```python
from build123d import *

# Parameters (mm, degrees)
SKETCH1_W   = 75
SKETCH1_H   = 250
SKETCH2_W   = 69.969867672
SKETCH2_H   = 30
SKETCH2_H_2 = 31.89416608
SKETCH2_H_3 = 30.244467835


with BuildPart() as part:
    # Sketch1 → Revolve1 (revolve)
    with BuildSketch(Plane.XY, mode=Mode.PRIVATE) as revolve1_sk:
        with Locations((-112.5, 125)):
            Rectangle(SKETCH1_W, SKETCH1_H)
    revolve(revolve1_sk.sketch.rotate(Axis((0, 0, 0), (0, 1, 0)), 270), axis=Axis((0, 0, 0), (0, 1, 0)))

    # Sketch2 → Cut-Revolve2 (revolve, cut)
    with BuildSketch(Plane.XY, mode=Mode.PRIVATE) as cut_revolve2_sk:
        with Locations((-115.015066164, 205)):
            Rectangle(SKETCH2_W, SKETCH2_H)
        with Locations((-115.015066164, 148.026485549)):
            Rectangle(SKETCH2_W, SKETCH2_H)
        with Locations((-115.015066164, 94.533526487)):
            Rectangle(SKETCH2_W, SKETCH2_H_2)
        with Locations((-115.015066164, 35.419339356)):
            Rectangle(SKETCH2_W, SKETCH2_H_3)
    revolve(cut_revolve2_sk.sketch.rotate(Axis((0, 0, 0), (0, 1, 0)), 180), axis=Axis((0, 0, 0), (0, 1, 0)), mode=Mode.SUBTRACT)


solid = part.part
```
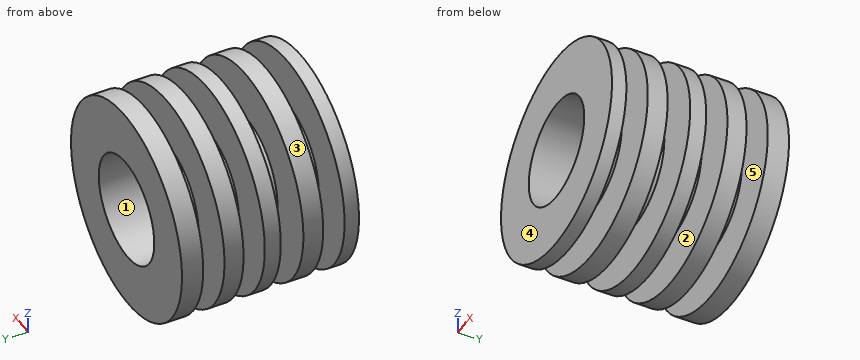
The model under review builds one solid part; all positions refer to its coordinate system, in mm. Face numbers are marked on the shaded views. A direction names the side the tool comes from. Coordinates: 2 decimals unless noted, no trailing zeros. Order: outer loops, then holes, each group sorted by start corner. A loop starts at its lowest first (then second) coordinate and runs counter-clockwise, first axis right, second up. Notation, with made-up numbers: (64.5, -8.75) -> (96.5, -8.75) arc R10 cw to (96.5, 5.25) -> close; hole circle Ø5 at (16.5, 6.5). An arc over 180 degrees is marked (long way). Answer in a Markdown table with one row per item. Add a question column.
Item 1: To check wall thickness, follow probe 1 along Y at (x, z) = (118.5, -73); probe 2 along X at (y, z) = (130.5, 0); probe 3 along X at (y, z) = (185, -30). State the ranges of each line that lie inside material, in increasing order.
Item 2: Clearance check with flat-ended pins moving along their axes: pin 1 (3 mm diameter, centred on y = 144, z = 28.5, fed in from +X); pin 2 (8 mm diameter, centred on y = 62, z = -106, fed in from +X); pin 3 (8 mm diameter, centred on x = 119.5, y = 191.5, fed in from -Z). State where each tip first meets the part, or that it passes through.
Item 3: We need section B-B on x = 115. Write out the cut boundary in (y, z).
Item 4: We need section A-A on z = 95. Write out the cut boundary in (x, y).
Item 5: Machinability: for the marked faces 4 and 5, which of the approach directions +Z, -Z, +X, -X, +Y, -Y give a long, thin tool a straight path to every point of the face, cutting with its end or side? Answer none if there is none.
Item 6: Mouldability with a two-part tool opening along X and no side actions: class the marked faces 1, 2 and 3 as +X half, -X half, draft (parallel to the pull), parting line (faces both ways), or undercut.
Item 7: We need section C-C on y = 215. Write out the cut boundary in (x, z), plus the area to 3 significant figures.
Final values:
| question | item | result |
|---|---|---|
| 1 | probe 1 | y = 0 to 20.3, 50.54 to 78.59, 110.48 to 133.03, 163.03 to 190, 220 to 250 |
| 1 | probe 2 | x = -150 to -75, 75 to 150 |
| 1 | probe 3 | x = -146.97 to -68.74, 68.74 to 146.97 |
| 2 | pin 1 | stops at x = 75.34 |
| 2 | pin 2 | stops at x = 109.98 |
| 2 | pin 3 | stops at z = -95.35 |
| 3 | outline | (0, -96.31) -> (20.3, -96.31) -> (20.3, 96.31) -> (0, 96.31) -> close; (50.54, -96.31) -> (78.59, -96.31) -> (78.59, 96.31) -> (50.54, 96.31) -> close; (110.48, -96.31) -> (133.03, -96.31) -> (133.03, 96.31) -> (110.48, 96.31) -> close; (163.03, -96.31) -> (190, -96.31) -> (190, 96.31) -> (163.03, 96.31) -> close; (220, -96.31) -> (250, -96.31) -> (250, 96.31) -> (220, 96.31) -> close |
| 4 | outline | (-116.08, 0) -> (116.08, 0) -> (116.08, 20.3) -> (-116.08, 20.3) -> close; (-116.08, 50.54) -> (116.08, 50.54) -> (116.08, 78.59) -> (-116.08, 78.59) -> close; (-116.08, 110.48) -> (116.08, 110.48) -> (116.08, 133.03) -> (-116.08, 133.03) -> close; (-116.08, 163.03) -> (116.08, 163.03) -> (116.08, 190) -> (-116.08, 190) -> close; (-116.08, 220) -> (116.08, 220) -> (116.08, 250) -> (-116.08, 250) -> close |
| 5 | face 4 | +Z, -Z, +X, -X, -Y |
| 5 | face 5 | none |
| 6 | face 1 | undercut |
| 6 | face 2 | draft |
| 6 | face 3 | parting line |
| 7 | outline | circle Ø160.06 at (0, 0); hole circle Ø150 at (0, 0) |
| 7 | area | 2,450 mm2 |
